from build123d import *

# Parameters (mm, degrees)
SKETCH2_W              = 30
SKETCH2_H              = 30
BOSS_EXTRUDE1_DEPTH    = 6
CUT_EXTRUDE1_START     = -1
CUT_EXTRUDE1_OUTLINE_W = 24
CUT_EXTRUDE1_OUTLINE_H = 24
CUT_EXTRUDE1_DEPTH     = 1
SKETCH4_W              = 24
SKETCH4_H              = 24
SKETCH4_R              = 6.5
CUT_EXTRUDE2_DEPTH     = 2
SKETCH5_W              = 3
SKETCH5_H              = 24
BOSS_EXTRUDE2_DEPTH    = 2
SKETCH6_W              = 24
SKETCH6_H              = 3
BOSS_EXTRUDE3_DEPTH    = 2
FILLET1_R              = 1
FILLET2_R              = 1
SKETCH8_R              = 1.25
CUT_EXTRUDE3_DEPTH     = 10
SKETCH7_R              = 1.25
CUT_EXTRUDE4_DEPTH     = 6
FILLET3_R              = 1
SKETCH10_R             = 10.5
BOSS_EXTRUDE4_DEPTH    = 9
SKETCH11_R             = 9
CUT_EXTRUDE5_DEPTH     = 3
SKETCH9_R              = 2.5
CUT_EXTRUDE6_DEPTH     = 26.416530054
SKETCH12_R             = 1
CUT_EXTRUDE7_DEPTH     = 13
SKETCH13_W             = 15.514513233
SKETCH13_H             = 2.095553254
CUT_EXTRUDE9_DEPTH     = 7
CHAMFER1_SIZE          = 1


# Read off the part's stored shape, not the designer's step: Cut-Extrude1
with BuildPart() as part:
    # Sketch2 → Boss-Extrude1 (new body)
    with BuildSketch(Plane.XY):
        Rectangle(SKETCH2_W, SKETCH2_H)
    extrude(amount=BOSS_EXTRUDE1_DEPTH)

    # Cut-Extrude1 outline → Cut-Extrude1 (cut)
    with BuildSketch(Plane.XY.offset(6).offset(CUT_EXTRUDE1_START)):
        Rectangle(CUT_EXTRUDE1_OUTLINE_W, CUT_EXTRUDE1_OUTLINE_H)
    extrude(amount=CUT_EXTRUDE1_DEPTH, mode=Mode.SUBTRACT)

    # Sketch4 → Cut-Extrude2 (cut)
    with BuildSketch(Plane.XY.offset(5)):
        Rectangle(SKETCH4_W, SKETCH4_H)
        Circle(SKETCH4_R, mode=Mode.SUBTRACT)
    extrude(amount=-CUT_EXTRUDE2_DEPTH, mode=Mode.SUBTRACT)

    # Sketch5 → Boss-Extrude2 (add)
    with BuildSketch(Plane.XY.offset(5)):
        Rectangle(SKETCH5_W, SKETCH5_H)
    extrude(amount=-BOSS_EXTRUDE2_DEPTH)

    # Sketch6 → Boss-Extrude3 (add)
    with BuildSketch(Plane.XY.offset(5)):
        Rectangle(SKETCH6_W, SKETCH6_H)
    extrude(amount=-BOSS_EXTRUDE3_DEPTH)

    # Fillet1
    fillet1_edges = [part.edges().sort_by_distance(p)[0] for p in [
        (1.5, 6.32455532, 4),
        (-1.5, -6.32455532, 4),
        (1.5, -6.32455532, 4),
        (-1.5, 6.32455532, 4),
        (6.32455532, -1.5, 4),
        (6.32455532, 1.5, 4),
        (-6.32455532, -1.5, 4),
        (-6.32455532, 1.5, 4),
    ]]
    fillet(fillet1_edges, radius=FILLET1_R)

    # Fillet2
    fillet2_edges = [part.edges().sort_by_distance(p)[0] for p in [
        (12, 12, 4.5),
        (12, -12, 4.5),
        (-12, -12, 4.5),
        (-12, 12, 4.5),
        (1.5, 12, 4),
        (-1.5, -12, 4),
        (1.5, -12, 4),
        (-1.5, 12, 4),
        (12, -1.5, 4),
        (12, 1.5, 4),
        (-12, -1.5, 4),
        (-12, 1.5, 4),
    ]]
    fillet(fillet2_edges, radius=FILLET2_R)

    # Sketch8 → Cut-Extrude3 (cut)
    with BuildSketch(Plane.XY.offset(3)):
        with Locations((-9.19, -9.19)):
            Circle(SKETCH8_R)
        with Locations((9.19, -9.19)):
            Circle(SKETCH8_R)
    extrude(amount=-CUT_EXTRUDE3_DEPTH, mode=Mode.SUBTRACT)

    # Sketch7 → Cut-Extrude4 (cut)
    with BuildSketch(Plane.XY.offset(6)):
        with Locations((-9.19, 9.19)):
            Circle(SKETCH7_R)
        with Locations((9.19, 9.19)):
            Circle(SKETCH7_R)
    extrude(amount=-CUT_EXTRUDE4_DEPTH, mode=Mode.SUBTRACT)

    # Fillet3
    fillet3_edges = [part.edges().sort_by_distance(p)[0] for p in [
        (15, -15, 3),
        (-15, -15, 3),
        (-15, 15, 3),
        (15, 15, 3),
    ]]
    fillet(fillet3_edges, radius=FILLET3_R)

    # Sketch10 → Boss-Extrude4 (add)
    with BuildSketch(Plane(origin=(0, 0, 0), x_dir=(-1, 0, 0), z_dir=(0, 0, -1))):
        Circle(SKETCH10_R)
    extrude(amount=BOSS_EXTRUDE4_DEPTH)

    # Sketch11 → Cut-Extrude5 (cut)
    with BuildSketch(Plane(origin=(0, 0, -9), x_dir=(-1, 0, 0), z_dir=(0, 0, -1))):
        Circle(SKETCH11_R)
    extrude(amount=-CUT_EXTRUDE5_DEPTH, mode=Mode.SUBTRACT)

    # Sketch9 → Cut-Extrude6 (cut, through all)
    with BuildSketch(Plane.XY.offset(5)):
        Circle(SKETCH9_R)
    extrude(amount=-CUT_EXTRUDE6_DEPTH, mode=Mode.SUBTRACT)

    # Sketch12 → Cut-Extrude7 (cut)
    with BuildSketch(Plane(origin=(0, 0, 0), x_dir=(-1, 0, 0), z_dir=(0, 0, -1))):
        with Locations((13, 13)):
            Circle(SKETCH12_R)
        with Locations((-13, 13)):
            Circle(SKETCH12_R)
        with Locations((-13, -13)):
            Circle(SKETCH12_R)
        with Locations((13, -13)):
            Circle(SKETCH12_R)
    extrude(amount=-CUT_EXTRUDE7_DEPTH, mode=Mode.SUBTRACT)

    # Sketch13 → Cut-Extrude9 (cut)
    with BuildSketch(Plane(origin=(0, 0, -9), x_dir=(-1, 0, 0), z_dir=(0, 0, -1))):
        with Locations((1.781437306, 10.347776627)):
            Rectangle(SKETCH13_W, SKETCH13_H)
    extrude(amount=-CUT_EXTRUDE9_DEPTH, mode=Mode.SUBTRACT)

    # Chamfer1
    chamfer1_edges = [part.edges().sort_by_distance(p)[0] for p in [
        (-2.5, 0, 5),
    ]]
    chamfer(chamfer1_edges, length=CHAMFER1_SIZE)


solid = part.part
Geometry: final body of the model. Coordinates: model frame, mm. A direction names the side the tool comes from. Round coordinates to 2 decimals unless told otherwise and drop trailing zeros. Loops run counter-clockwise (first coordinate to the right, second up) from the corner with the lowest first, then second, coordinate; pieces in that order, holes last. Notation, with made-up numbers: (62, -23.5) - (75, -23.5) arc R3 cw to (75, -18.5) - close; hole circle Ø5 at (54.5, 79.25). An arc over 180 degrees is marked (long way). Write each question's results on one line, items separated by ' | '. Start each with the question number.
1) Line query: probe 1 along Y at (x, z) = (9.19, 1.2); probe 2 along Y at (x, z) = (-13, 1.45); probe 3 along X at (y, z) = (13.25, 0.25). Output: solid intervals per line, ascending. Write a range as [from, to].
2) Access query for faces 5 (the face through (-15, 0, 3)), 6 (the face through (1.172, 8.923, -7.521)), 7 (the face through (-7, 7, 3)). Directions: +Z, -Z, +X, -X, +Y, -Y. A direction counts if a zero-diameter tool reaches every point of the face in a straight line with its end or side. Return the directions, or none.
3) Cut plane B-B on y = 0. Return loops of the section in (x, z).
4) Mould query, pull axis Y, two halves, no side actions, for faces 1 (the face through (9.862, 10.244, 1.521)), 2 (the face through (-4.845, -9.315, -4.437)), 3 (the face through (0, 15, 3)), 4 (the face through (-14.715, -14.699, 3.042)). Classes: released by +Y, released by -Y, zero draft, split by the parting line, or undercut.
5) First-contact query: P1, Ø8, axis at y = -11.5, z = -5, coming from the +X side; P2, Ø8, axis at x = 0, y = 0, coming from the -Z side; P3, Ø3, axis at x = -9.19, y = 9.19, coming from the -Z side; P4, Ø2, axis at x = 9.19, y = -9.19, coming from the -Z side. Flat tips, straight axial feed; report the tip coordinate or a pass-through.
6) Cut plane C-C on x = 13. Return loops of the section in (y, z), then the cut area to 3 significant figures.
7) Cut plane A-A on x = 0. Return loops of the section in (y, z).
8) Cut plane D-D on z = 2. Count the separate pieces of the cut face and the enclosed holes in it, then the cut area to 3 significant figures.
Verdict:
1) probe 1: y = [-15, -10.44], [-7.94, 7.94], [10.44, 15] | probe 2: y = [-15, -14], [-12, 12], [14, 15] | probe 3: x = [-15, -13.97], [-12.03, 12.03], [13.97, 15]
2) face 5: +Z, -Z, -X, +Y, -Y | face 6: -Z | face 7: +Z
3) outline: (-15, 0) - (-10.5, 0) - (-10.5, -9) - (-9, -9) - (-9, -6) - (-2.5, -6) - (-2.5, 4) - (-3.5, 5) - (-12, 5) - (-12, 6) - (-15, 6) - close; (2.5, -6) - (9, -6) - (9, -9) - (10.5, -9) - (10.5, 0) - (15, 0) - (15, 6) - (12, 6) - (12, 5) - (3.5, 5) - (2.5, 4) - close
4) face 1: undercut | face 2: split by the parting line | face 3: released by +Y | face 4: released by -Y
5) P1: stops at x = 7.35 | P2: stops at z = -6 | P3: stops at z = 0 | P4: passes through
6) outline: (-15, 0) - (-14, 0) - (-14, 6) - (-15, 6) - close; (-12, 0) - (12, 0) - (12, 6) - (-12, 6) - close; (14, 0) - (15, 0) - (15, 6) - (14, 6) - close | area: 156 mm2
7) outline: (-15, 0) - (-10.5, 0) - (-10.5, -9) - (-9, -9) - (-9, -6) - (-2.5, -6) - (-2.5, 4) - (-3.5, 5) - (-12, 5) - (-12, 6) - (-15, 6) - close; (2.5, -6) - (9, -6) - (9, -9) - (9.3, -9) - (9.3, -2) - (10.5, -2) - (10.5, 0) - (15, 0) - (15, 6) - (12, 6) - (12, 5) - (3.5, 5) - (2.5, 4) - close
8) separate pieces: 1 | enclosed holes: 9 | area: 847 mm2
